from build123d import *

# Parameters (mm, degrees)
SKETCH1_R           = 1.4
SKETCH1_W           = 43.5
SKETCH1_H           = 21
BOSS_EXTRUDE1_DEPTH = 5
CHAMFER1_SIZE       = 3
CHAMFER1_SIZE2      = 1.732050808
SKETCH3_R           = 1.4
CUT_EXTRUDE2_DEPTH  = 148.599330961
SKETCH5_R           = 3
BOSS_EXTRUDE2_DEPTH = 5
SKETCH6_R           = 1.4
CUT_EXTRUDE3_DEPTH  = 148.59933107


with BuildPart() as part:
    # Sketch1 → Boss-Extrude1 (new body)
    with BuildSketch(Plane(origin=(0, 0, 0), x_dir=(1, 0, 0), z_dir=(0, 1, 0))):
        with BuildLine():
            Line((0, 15), (131.75, 15))
            ThreePointArc((131.75, 15), (146.75, 0), (131.75, -15))
            Line((131.75, -15), (0, -15))
            ThreePointArc((0, -15), (-15, 0), (0, 15))
        make_face()
        with Locations(Location((0, 0, 0), (0, 0, 270))):
            Circle(SKETCH1_R, mode=Mode.SUBTRACT)
        with Locations(Location((85.5, 5, 0), (0, 0, 270))):
            Circle(SKETCH1_R, mode=Mode.SUBTRACT)
        with Locations(Location((85.5, -5, 0), (0, 0, 90))):
            Circle(SKETCH1_R, mode=Mode.SUBTRACT)
        with Locations(Location((134.5, -5, 0), (0, 0, 270))):
            Circle(SKETCH1_R, mode=Mode.SUBTRACT)
        with Locations(Location((134.5, 5, 0), (0, 0, 90))):
            Circle(SKETCH1_R, mode=Mode.SUBTRACT)
        with Locations((110, 0)):
            Rectangle(SKETCH1_W, SKETCH1_H, mode=Mode.SUBTRACT)
    extrude(amount=BOSS_EXTRUDE1_DEPTH)

    # Chamfer1
    chamfer1_edges = [part.edges().sort_by_distance(p)[0] for p in [
        (65.875, 0, -15),
        (146.75, 0, 0),
        (65.875, 0, 15),
        (-15, 0, 0),
    ]]
    chamfer1_side = [part.faces().sort_by_distance(p)[0] for p in [
        (54.841734093, 0, 0),
    ]]
    chamfer(chamfer1_edges, length=CHAMFER1_SIZE, length2=CHAMFER1_SIZE2, reference=chamfer1_side[0])

    # Sketch3 → Cut-Extrude2 (cut, through all)
    with BuildSketch(Plane.XZ):
        with Locations(Location((76.75, 5, 0), (0, 0, 270))):
            Circle(SKETCH3_R)
        with Locations(Location((76.75, -5, 0), (0, 0, 90))):
            Circle(SKETCH3_R)
    extrude(amount=-CUT_EXTRUDE2_DEPTH, mode=Mode.SUBTRACT)

    # Sketch5 → Boss-Extrude2 (add)
    with BuildSketch(Plane.XZ):
        with Locations((142.658712115, -5)):
            Circle(SKETCH5_R)
    boss_extrude2 = extrude(amount=-BOSS_EXTRUDE2_DEPTH)

    # Sketch6 → Cut-Extrude3 (cut, through all)
    with BuildSketch(Plane.XZ):
        with Locations(Location((142.658712115, -5, 0), (0, 0, 270))):
            Circle(SKETCH6_R)
    cut_extrude3 = extrude(amount=-CUT_EXTRUDE3_DEPTH, mode=Mode.SUBTRACT)

    # Mirror1: Boss-Extrude2, Cut-Extrude3 across plane
    add(boss_extrude2.mirror(Plane.XY))
    add(cut_extrude3.mirror(Plane.XY), mode=Mode.SUBTRACT)


solid = part.part
Could you check a few things on this model? Use its own coordinates, in mm. A direction names the side the tool comes from. Give positions to 0.01 mm unless a question says otherwise; leave off trailing zeros. Write each loop counter-clockwise with the first axis right and the second up, starting at its lowest first coordinate (ties: lowest second). Pieces come first, ordered by that corner, then holes. Notation, with made-up numbers: (33, 28) -> (65, 28) arc R5 ccw to (65, 32) -> close; hole circle Ø1 at (32, 24). An arc over 180 degrees is marked (long way). Answer as a JSON object with one key per item and string values.
Q1. Which directions (+Z, -Z, +X, -X, +Y, -Y) give clear straight access to the entire face, cutting with the end or side of a thin tool? Please do faces 1 (the flat face through (110, 2, -10.5)), 2 (the cylindrical face through (145.355, 0.661, -6.314)), 3 (the flat face through (66.797, 0.878, 13.521)).
Taken from the geometry:
{"face 1": "+Y, -Y", "face 2": "-Y", "face 3": "+Z, +X, -X, -Y"}
Q2. Suppose I cut it at A-A on x = 76.75. Write out the boundary of the cut face in (y, z), then the cut area to 3 significant figures.
Taken from the geometry:
{"outline": "(0, -12) -> (1.73, -15) -> (5, -15) -> (5, -6.4) -> (0, -6.4) -> close; (0, -3.6) -> (5, -3.6) -> (5, 3.6) -> (0, 3.6) -> close; (0, 6.4) -> (5, 6.4) -> (5, 15) -> (1.73, 15) -> (0, 12) -> close", "area": "117 mm²"}
Q3. We'd pull the mould along X, two halves only. Please class faces 4 (the cylindrical face through (141.42, 2.46, 5.65)), 5 (the cylindrical face through (-15, 3, 0)), 6 (the flat face through (48, 0, 0)), 7 (the cylindrical face through (84.133, 2.465, -5.303)): released by +X, released by -X, zero draft, split by the parting line, or undercut.
Taken from the geometry:
{"face 4": "undercut", "face 5": "released by -X", "face 6": "zero draft", "face 7": "undercut"}
Q4. Will these pins go through, and if not, where does the flat tip stop? pin 1 Ø1 at (y, z) = (4.5, -8) entering from -X; pin 2 Ø1 at (x, y) = (14, 1) entering from +Z; pin 3 Ø1.5 at (y, z) = (2.5, 1.5) entering from +X.
Taken from the geometry:
{"pin 1": "stops at x = -12.99", "pin 2": "stops at z = 14.6", "pin 3": "stops at x = 146.73"}
Q5. Please list where these lines run through material, in increasing order: L1, parallel to Z at x = 76.75, y = 1.85; L2, parallel to Z at x = 128, y = 1.9; L3, parallel to X at y = 1.5, z = -5.
Taken from the geometry:
{"L1": "z = -15 to -6.4, -3.6 to 3.6, 6.4 to 15", "L2": "z = -15 to -10.5, 10.5 to 15", "L3": "x = -13.72 to 75.35, 78.15 to 84.1, 86.9 to 88.25, 131.75 to 133.1, 135.9 to 141.26, 144.06 to 145.66"}
Q6. Suppose I cut it at C-C on y = 3.55. Count the separate pieces of the cut face and the enclosed holes in it, then the cut area to 3 significant figures.
Taken from the geometry:
{"separate pieces": "1", "enclosed holes": "10", "area": "3,690 mm²"}
Q7. Suppose I cut it at B-B on x = 128.5. Write out the boundary of the cut face in (y, z).
Taken from the geometry:
{"outline": "(0, -12) -> (1.73, -15) -> (5, -15) -> (5, -10.5) -> (0, -10.5) -> close; (0, 10.5) -> (5, 10.5) -> (5, 15) -> (1.73, 15) -> (0, 12) -> close"}
